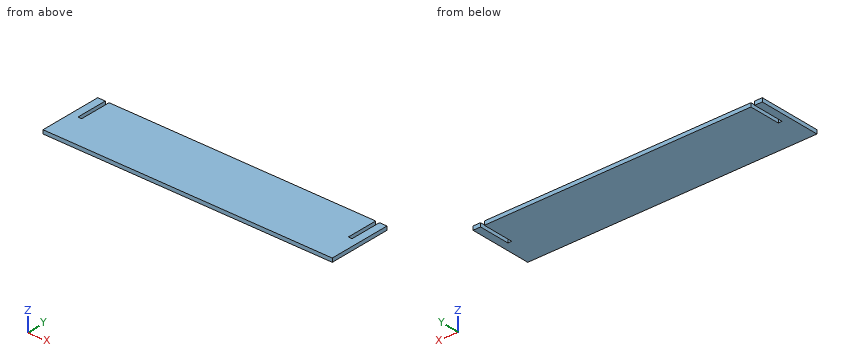
from build123d import *

# Parameters (mm, degrees)
BOSS_EXTRU_1_DEPTH = 3


with BuildPart() as part:
    # Esquisse1 → Boss.-Extru.1 (new body)
    with BuildSketch(Plane.XY):
        Polygon((-109, 25), (-109, 0), (-106, 0), (-106, 25), (106, 25), (106, 0), (109, 0), (109, 25), (115, 25), (115, -25), (-115, -25), (-115, 25), align=None)
    extrude(amount=BOSS_EXTRU_1_DEPTH)


solid = part.part
Could you check a few things on this model? Use its own coordinates, in mm. Give positions to 0.01 mm unless a question says otherwise; leave off trailing zeros. Order: outer loops, then holes, each group sorted by start corner. A loop starts at its lowest first (then second) coordinate and runs counter-clockwise, first axis right, second up. Notation, with made-up numbers: (-10.5, -8.75) -> (43.5, -8.75) arc R21 cw to (43.5, 17.25) -> close; hole circle Ø5 at (2, 38.25). An arc over 180 degrees is marked (long way). Return JSON: item names as keys, results as strings.
1. For pin 1 Ø0.9 at (x, z) = (107, 2) entering from +Y; pin 2 Ø3 at (x, y) = (20.5, -18.5) entering from -Z, each with a flat end and sliding along its axis, tell me the tip position at first contact or that it passes through.
Answer list:
{"pin 1": "stops at y = 0", "pin 2": "stops at z = 0"}
2. Imagine slicing it at A-A on y = 5.5. List the corners of the cut face in (x, z) for me, then the cut area to 3 significant figures.
Answer list:
{"outline": "(-115, 0) -> (-109, 0) -> (-109, 3) -> (-115, 3) -> close; (-106, 0) -> (106, 0) -> (106, 3) -> (-106, 3) -> close; (109, 0) -> (115, 0) -> (115, 3) -> (109, 3) -> close", "area": "672 mm2"}
3. I need wall thicknesses on line 1 (X direction, y = 0.5, z = 0.4). Which ranges of the line are inside material? Lowest first, please. Write a range as from..to.
Answer list:
{"line 1": "x = -115..-109, -106..106, 109..115"}
